Can you work these out from the model? Positions are in its coordinate system, mm. A direction names the side the tool comes from. Coordinates: 2 decimals unless noted, no trailing zeros. Write each loop counter-clockwise with the first axis right and the second up, starting at its lowest first coordinate (ties: lowest second). Pieces come first, ordered by that corner, then holes. Notation, with made-up numbers: (36.5, 45) -> (95.5, 45) arc R28 ccw to (95.5, 82) -> close; hole circle Ø10 at (-24.75, 81). An arc over 180 degrees is marked (long way). Use one line per item in the form item = value.
```python
from build123d import *

# Parameters (mm, degrees)
F1_DEPTH = 1828.8
F4_D     = 19.05
F5_D     = 12.7


with BuildPart() as f1:
    # F0 (on Front) → F1 (new body)
    with BuildSketch(Plane.XZ):
        Polygon((6.35, 152.4), (-6.35, 152.4), (-6.35, 0), (0, 0), (6.35, 0), (146.05, 0), (146.05, 12.7), (6.35, 12.7), align=None)
    extrude(amount=F1_DEPTH)

    # F4 (through all)
    with Locations(Plane(origin=(0, 0, 0), x_dir=(1, 0, 0), z_dir=(0, 0, -1))):
        with Locations((69.85, 1066.8), (69.85, 1219.2), (69.85, 1371.6), (69.85, 1524), (69.85, 1676.4), (69.85, 914.4), (69.85, 762), (69.85, 609.6), (69.85, 457.2), (69.85, 304.8), (69.85, 152.4)):
            Hole(F4_D / 2)

    # F5 (through all)
    with Locations(Plane(origin=(-6.35, 0, 0), x_dir=(0, -1, 0), z_dir=(-1, 0, 0))):
        with Locations((1600.2, 76.2), (1371.6, 76.2), (1143, 76.2), (914.4, 76.2), (685.8, 76.2), (457.2, 76.2), (228.6, 76.2)):
            Hole(F5_D / 2)


solid = f1.part
```
Q1. If I drill on line 1 (Z direction, x = -0.25, y = -1143); line 2 (X direction, y = -1676, z = 6); line 3 (Z direction, x = 66.5, y = -1246), over which ranges is the centre line in solid material (lowest first)? Write a range as from..to.
Return value:
line_1 = 0..69.85, 82.55..152.4
line_2 = -6.35..60.33, 79.37..146.05
line_3 = 0..12.7
Q2. Suppose I cut it at B-B (x = 106.5). Write out the boundary of the cut face in (y, z).
Return value:
outline = (-1828.8, 0) -> (0, 0) -> (0, 12.7) -> (-1828.8, 12.7) -> close
Q3. For faces 1 (the flat face through (2, 0, 43)), 2 (the flat face through (6.35, -902, 82)), which set-ups out of +Z, -Z, +X, -X, +Y, -Y let a thin tool reach every point of the face, with its end or its side?
Return value:
face_1 = +Z, -Z, +X, -X, +Y
face_2 = +Z, +X, +Y, -Y
Q4. Suppose I cut it at C-C (z = 102). Write out the boundary of the cut face in (x, y), then the cut area to 3 significant figures.
Return value:
outline = (-6.35, -1828.8) -> (6.35, -1828.8) -> (6.35, 0) -> (-6.35, 0) -> close
area = 23,200 mm2
Q5. Will these pins go through, and if not, where does the flat tip stop? pin 1 (11.5 mm diameter, centred on x = 69.85, y = -1371.6, fed in from -Z); pin 2 (14.5 mm diameter, centred on y = -1371.6, z = 76.2, fed in from +X); pin 3 (25 mm diameter, centred on x = 69.85, y = -762, fed in from +Z).
Return value:
pin_1 = through
pin_2 = 6.35
pin_3 = 12.7
Q6. Suppose I cut it at A-A (y = -1480). Write out the boundary of the cut face in (x, z), then the cut area to 3 significant figures.
Return value:
outline = (-6.35, 0) -> (146.05, 0) -> (146.05, 12.7) -> (6.35, 12.7) -> (6.35, 152.4) -> (-6.35, 152.4) -> close
area = 3,710 mm2
